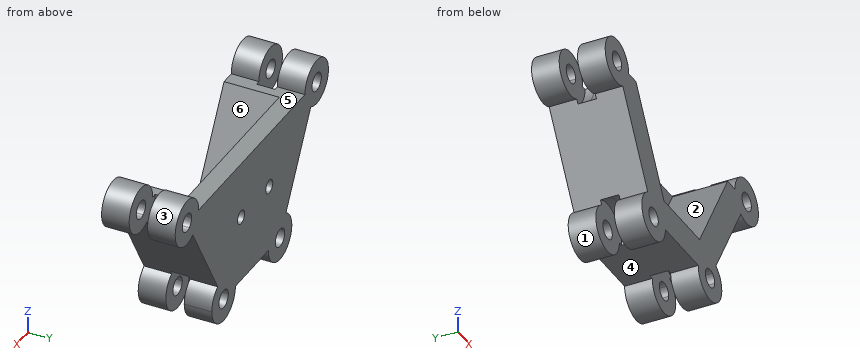
```python
from build123d import *

# Parameters (mm, degrees)
F1_DEPTH = 50.8
F3_DEPTH = 76.2
F4_R     = 38.1
F5_DEPTH = 12.7
F6_R     = 9.525
F7_DEPTH = 25.401


with BuildPart() as f1:
    # F0 (on Front) → F1 (new body, symmetric)
    with BuildSketch(Plane.XZ):
        with BuildLine():
            ThreePointArc((-83.1071616711, -65.430798607), (-83.1071616711, -120.4234117473), (-35.4821616711, -92.9271051772))
            Line((-35.4821616711, -92.9271051772), (-54.5321616711, -92.9271051772))
            ThreePointArc((-54.5321616711, -92.9271051772), (-73.5821616711, -103.9256278052), (-73.5821616711, -81.9285825491))
            Line((-73.5821616711, -81.9285825491), (-83.1071616711, -65.430798607))
        make_face()
        with BuildLine():
            ThreePointArc((-83.1071616711, -65.430798607), (-51.3571616711, -65.430798607), (-35.4821616711, -92.9271051772))
            Line((-35.4821616711, -92.9271051772), (53.4178383289, -92.9271051772))
            ThreePointArc((53.4178383289, -92.9271051772), (69.2928383289, -65.430798607), (101.0428383289, -65.430798607))
            Line((101.0428383289, -65.430798607), (168.2795419814, 51.0265882527))
            ThreePointArc((168.2795419814, 51.0265882527), (156.6582354113, 62.6478948228), (152.4045419814, 78.5228948228))
            Line((152.4045419814, 78.5228948228), (-134.4688653237, 78.5228948228))
            ThreePointArc((-134.4688653237, 78.5228948228), (-138.7225587535, 62.6478948228), (-150.3438653237, 51.0265882527))
            Line((-150.3438653237, 51.0265882527), (-83.1071616711, -65.430798607))
        make_face()
        with BuildLine():
            Line((-54.5321616711, -92.9271051772), (-35.4821616711, -92.9271051772))
            ThreePointArc((-35.4821616711, -92.9271051772), (-51.3571616711, -65.430798607), (-83.1071616711, -65.430798607))
            Line((-83.1071616711, -65.430798607), (-73.5821616711, -81.9285825491))
            ThreePointArc((-73.5821616711, -81.9285825491), (-60.8821616711, -81.9285825491), (-54.5321616711, -92.9271051772))
        make_face()
        with BuildLine():
            ThreePointArc((101.0428383289, -65.430798607), (69.2928383289, -65.430798607), (53.4178383289, -92.9271051772))
            Line((53.4178383289, -92.9271051772), (72.4678383289, -92.9271051772))
            ThreePointArc((72.4678383289, -92.9271051772), (78.8178383289, -81.9285825491), (91.5178383289, -81.9285825491))
            Line((91.5178383289, -81.9285825491), (101.0428383289, -65.430798607))
        make_face()
        with BuildLine():
            Line((72.4678383289, -92.9271051772), (53.4178383289, -92.9271051772))
            ThreePointArc((53.4178383289, -92.9271051772), (85.1678383289, -124.6771051772), (116.9178383289, -92.9271051772))
            ThreePointArc((116.9178383289, -92.9271051772), (112.664144899, -77.0521051772), (101.0428383289, -65.430798607))
            Line((101.0428383289, -65.430798607), (91.5178383289, -81.9285825491))
            ThreePointArc((91.5178383289, -81.9285825491), (96.1663609569, -86.5771051772), (97.8678383289, -92.9271051772))
            ThreePointArc((97.8678383289, -92.9271051772), (85.1678383289, -105.6271051772), (72.4678383289, -92.9271051772))
        make_face()
        with BuildLine():
            ThreePointArc((-134.4688653237, 78.5228948228), (-193.7151718938, 94.3978948228), (-150.3438653237, 51.0265882527))
            Line((-150.3438653237, 51.0265882527), (-159.8688653237, 67.5243721948))
            ThreePointArc((-159.8688653237, 67.5243721948), (-177.2173879518, 84.8728948228), (-153.5188653237, 78.5228948228))
            Line((-153.5188653237, 78.5228948228), (-134.4688653237, 78.5228948228))
        make_face()
        with BuildLine():
            Line((-159.8688653237, 67.5243721948), (-150.3438653237, 51.0265882527))
            ThreePointArc((-150.3438653237, 51.0265882527), (-138.7225587535, 62.6478948228), (-134.4688653237, 78.5228948228))
            Line((-134.4688653237, 78.5228948228), (-153.5188653237, 78.5228948228))
            ThreePointArc((-153.5188653237, 78.5228948228), (-155.2203426956, 72.1728948228), (-159.8688653237, 67.5243721948))
        make_face()
        with BuildLine():
            ThreePointArc((152.4045419814, 78.5228948228), (156.6582354113, 62.6478948228), (168.2795419814, 51.0265882527))
            Line((168.2795419814, 51.0265882527), (177.8045419814, 67.5243721948))
            ThreePointArc((177.8045419814, 67.5243721948), (173.1560193534, 72.1728948228), (171.4545419814, 78.5228948228))
            Line((171.4545419814, 78.5228948228), (152.4045419814, 78.5228948228))
        make_face()
        with BuildLine():
            Line((177.8045419814, 67.5243721948), (168.2795419814, 51.0265882527))
            ThreePointArc((168.2795419814, 51.0265882527), (200.0295419814, 51.0265882527), (215.9045419814, 78.5228948228))
            ThreePointArc((215.9045419814, 78.5228948228), (184.1545419814, 110.2728948228), (152.4045419814, 78.5228948228))
            Line((152.4045419814, 78.5228948228), (171.4545419814, 78.5228948228))
            ThreePointArc((171.4545419814, 78.5228948228), (184.1545419814, 91.2228948228), (196.8545419814, 78.5228948228))
            ThreePointArc((196.8545419814, 78.5228948228), (190.5045419814, 67.5243721948), (177.8045419814, 67.5243721948))
        make_face()
    extrude(amount=F1_DEPTH, both=True)

    # F2 (on face) → F3 (cut)
    with BuildSketch(Plane.XZ.offset(50.8)):
        Polygon((132.8281030505, 78.5228948228), (-114.8924263927, 78.5228948228), (-39.0819515524, -52.7846993466), (57.0176282101, -52.7846993466), align=None)
    extrude(amount=-F3_DEPTH, mode=Mode.SUBTRACT)

    # F4 (on Front) → F5 (cut, symmetric)
    with BuildSketch(Plane.XZ):
        with Locations((-166.2188653237, 78.5228948228)):
            Circle(F4_R)
        with Locations((-67.2321616711, -92.9271051772)):
            Circle(F4_R)
        with Locations((85.1678383289, -92.9271051772)):
            Circle(F4_R)
        with Locations((184.1545419814, 78.5228948228)):
            Circle(F4_R)
    extrude(amount=F5_DEPTH, both=True, mode=Mode.SUBTRACT)

    # F6 (on face) → F7 (cut, through all)
    with BuildSketch(Plane.XZ.offset(-25.4)):
        with Locations((-38.1, 0)):
            Circle(F6_R)
        with Locations((38.1, 0)):
            Circle(F6_R)
    extrude(amount=-F7_DEPTH, mode=Mode.SUBTRACT)


solid = f1.part
```
Source: CAD feature listing. Evaluate the final solid. Frame: model axes, mm. Face numbers are marked on the shaded views. A direction names the side the tool comes from. Give positions to 0.01 mm unless a question says otherwise; leave off trailing zeros. Write each loop counter-clockwise with the first axis right and the second up, starting at its lowest first coordinate (ties: lowest second). Pieces come first, ordered by that corner, then holes.
1. First-contact query: pin 1 (12 mm diameter, centred on y = -16.5, z = 51, fed in from -X); pin 2 (4 mm diameter, centred on x = -9.5, y = -34.5, fed in from -Z); pin 3 (5 mm diameter, centred on y = -14, z = 57, fed in from -X). Flat tips, straight axial feed; report the tip coordinate or a pass-through.
2. Section query D-D (x = 108.5). Return the cut outline in (y, z).
3. Pull-direction query (Z, two-part tool) for the marked faces 1, 2 and 3; classes: +Z half, -Z half, draft (parallel to the pull), parting line (faces both ways), or undercut.
4. Access query for the marked faces 4, 5 and 6. Directions: +Z, -Z, +X, -X, +Y, -Y. A direction counts if a zero-diameter tool reaches every point of the face in a straight line with its end or side. Return the directions, or none.
5. Material intervals for line 1 along Z through (x, y) = (38.1, 41.5) (3 decimals); line 2 along Z through (x, y) = (-38.1, 34) (3 decimals); line 3 along Y through (x, z) = (-87.5, -80), sorted ascending.
6. Section query C-C (y = 43.5). Return the cut outline in (x, z) (3 decimals), then the cut area to 3 significant figures.
7. Section query A-A (x = 38.1). Return the cut outline in (y, z) (3 decimals), then the cut area to 3 significant figures.
8. Section query B-B (z = 0). Return the cut outline in (x, y) (3 decimals).
Output values:
1. pin 1: stops at x = -189.56
1. pin 2: stops at z = -92.93
1. pin 3: stops at x = -191.64
2. outline: (-50.8, -114.46) - (-12.7, -114.46) - (-12.7, -71.39) - (-50.8, -71.39) - close; (-50.8, -52.51) - (50.8, -52.51) - (50.8, 78.52) - (25.4, 78.52) - (25.4, 36.39) - (-50.8, 36.39) - close; (12.7, -114.46) - (50.8, -114.46) - (50.8, -71.39) - (12.7, -71.39) - close
3. face 1: undercut
3. face 2: +Z half
3. face 3: parting line
4. face 4: -Z, +Y, -Y
4. face 5: +Z, +Y, -Y
4. face 6: +Z, -Y
5. line 1: z = -92.927 to -9.525, 9.525 to 78.523
5. line 2: z = -105.552 to -9.525, 9.525 to 78.523
5. line 3: y = -50.8 to -12.7, 12.7 to 50.8
6. outline: (-150.344, 51.027) - (-83.107, -65.431) arc R31.75 ccw (long way) to (-35.482, -92.927) - (53.418, -92.927) arc R31.75 ccw (long way) to (101.043, -65.431) - (168.28, 51.027) arc R31.75 ccw (long way) to (152.405, 78.523) - (-134.469, 78.523) arc R31.75 ccw (long way) to start; hole circle Ø25.4 at (-166.219, 78.523); hole circle Ø25.4 at (-67.232, -92.927); hole circle Ø19.05 at (-38.1, 0); hole circle Ø19.05 at (38.1, 0); hole circle Ø25.4 at (85.168, -92.927); hole circle Ø25.4 at (184.155, 78.523)
6. area: 50,000 mm2
7. outline: (-50.8, -92.927) - (50.8, -92.927) - (50.8, -9.525) - (25.4, -9.525) - (25.4, -52.785) - (-50.8, -52.785) - close; (25.4, 9.525) - (50.8, 9.525) - (50.8, 78.523) - (25.4, 78.523) - close
7. area: 6,930 mm2
8. outline: (-120.884, -50.8) - (-69.557, -50.8) - (-69.557, 25.4) - (-47.625, 25.4) - (-47.625, 50.8) - (-120.884, 50.8) - close; (-28.575, 25.4) - (28.575, 25.4) - (28.575, 50.8) - (-28.575, 50.8) - close; (47.625, 25.4) - (87.493, 25.4) - (87.493, -50.8) - (138.819, -50.8) - (138.819, 50.8) - (47.625, 50.8) - close
